```python
from build123d import *

# Parameters (mm, degrees)
F0_W     = 50.8
F0_H     = 431.8
F1_DEPTH = 25.4
F4_D     = 5.1054
F6_D     = 5.1054
F8_D     = 5.1054
F2_W     = 45.72
F2_H     = 20.32
F9_DEPTH = 431.8
F10_D    = 28.575


# Not quite as in the source:
# - a feature names something its author has since deleted; it is built from what else it names


with BuildPart() as f1:
    # F0 (on Top) → F1 (new body)
    with BuildSketch(Plane.XY):
        with Locations((-28.1036759261, 229.4025395081)):
            Rectangle(F0_W, F0_H)
    extrude(amount=F1_DEPTH)

    # F4 (through all)
    with Locations(Plane(origin=(-53.5036759261, 0, 0), x_dir=(0, -1, 0), z_dir=(-1, 0, 0))):
        with Locations((-26.2025395081, 12.7), (-331.0025395081, 12.7), (-381.8025395081, 12.7), (-356.4025395081, 12.7), (-407.2025395081, 12.7), (-178.6025395081, 12.7), (-229.4025395081, 12.7), (-204.0025395081, 12.7), (-280.2025395081, 12.7), (-254.8025395081, 12.7), (-305.6025395081, 12.7), (-102.4025395081, 12.7), (-153.2025395081, 12.7), (-51.6025395081, 12.7), (-127.8025395081, 12.7), (-77.0025395081, 12.7), (-432.6025395081, 12.7)):
            Hole(F4_D / 2)

    # F6 (through all)
    with Locations(Plane.XY.offset(25.4)):
        with Locations((-40.8036759261, 432.6025395081), (-15.4036759261, 432.6025395081), (-40.8036759261, 356.4025395081), (-40.8036759261, 381.8025395081), (-40.8036759261, 407.2025395081), (-40.8036759261, 254.8025395081), (-15.4036759261, 356.4025395081), (-15.4036759261, 254.8025395081), (-15.4036759261, 127.8025395081), (-40.8036759261, 102.4025395081), (-15.4036759261, 407.2025395081), (-15.4036759261, 331.0025395081), (-15.4036759261, 305.6025395081), (-40.8036759261, 204.0025395081), (-40.8036759261, 305.6025395081), (-15.4036759261, 280.2025395081), (-40.8036759261, 127.8025395081), (-15.4036759261, 381.8025395081), (-40.8036759261, 77.0025395081), (-40.8036759261, 178.6025395081), (-40.8036759261, 280.2025395081), (-15.4036759261, 77.0025395081), (-15.4036759261, 204.0025395081), (-15.4036759261, 178.6025395081), (-15.4036759261, 229.4025395081), (-15.4036759261, 153.2025395081), (-40.8036759261, 331.0025395081), (-40.8036759261, 229.4025395081), (-15.4036759261, 102.4025395081), (-40.8036759261, 153.2025395081)):
            Hole(F6_D / 2)

    # F8 (through all)
    with Locations(Plane.XY.offset(25.4)):
        with Locations((-45.6296759261, 56.4285395081), (-10.5776759261, 56.4285395081), (-10.5776759261, 21.3765395081), (-45.6296759261, 21.3765395081)):
            Hole(F8_D / 2)

    # F2 (on face) → F9 (cut)
    with BuildSketch(Plane(origin=(0, 445.3025395081, 0), x_dir=(-1, 0, 0), z_dir=(0, 1, 0))):
        with Locations((28.1036759261, 12.7)):
            Rectangle(F2_W, F2_H)
    extrude(amount=-F9_DEPTH, mode=Mode.SUBTRACT)

    # F10 (through all)
    with Locations(Plane.XY.offset(25.4)):
        with Locations((-28.1036759261, 38.9025395081)):
            Hole(F10_D / 2)


solid = f1.part
```
Here's how the part is built. I have some questions about the finished solid (model axes, mm). A direction names the side the tool comes from. Give positions to 0.01 mm unless a question says otherwise; leave off trailing zeros. Write each loop counter-clockwise with the first axis right and the second up, starting at its lowest first coordinate (ties: lowest second). Pieces come first, ordered by that corner, then holes.
(1) Imagine slicing it at B-B, the plane x = -34. Write out the boundary of the cut face in (y, z), and give its area (3 significant figures).
Output values:
outline: (13.5, 0) - (25.89, 0) - (25.89, 2.54) - (13.5, 2.54) - close; (13.5, 22.86) - (25.89, 22.86) - (25.89, 25.4) - (13.5, 25.4) - close; (51.92, 0) - (445.3, 0) - (445.3, 2.54) - (51.92, 2.54) - close; (51.92, 22.86) - (445.3, 22.86) - (445.3, 25.4) - (51.92, 25.4) - close
area: 2,060 mm2
(2) On a 3-axis mill with a long thin cutter (end or side, diameter ignored), from which of +Z, -Z, +X, -X, +Y, -Y can I reach the whole of each face in a straight line? I mean faces 4 (the face through (-53.504, 226, 13)), 5 (the face through (-50.964, 232.4, 12.6)). Say none if no direction works.
Output values:
face 4: +Z, -Z, -X, +Y, -Y
face 5: +Y, -Y
(3) If I drill on L1, parallel to X at y = 103, z = 23.5; L2, parallel to X at y = 222, z = 12.5; L3, parallel to Z at x = -24, y = 362, over which ranges is the centre line in solid material (lowest first)?
Output values:
L1: x = -53.5 to -43.29, -38.32 to -17.89, -12.92 to -2.7
L2: x = -53.5 to -50.96, -5.24 to -2.7
L3: z = 0 to 2.54, 22.86 to 25.4
(4) Thinking about a two-plate mould opening in X: for faces 1 (the face through (-28, 232, 25.4)), 2 (the face through (-2.704, 226, 13)), 3 (the face through (-28, 232, 22.86)), which applies, pulls with the +X half, pulls with the -X half, needs draft (parallel to the pull), parting line crosses it, or undercut?
Output values:
face 1: needs draft
face 2: pulls with the +X half
face 3: undercut
(5) Imagine slicing it at A-A, the plane y = 110. Write out the boundary of the cut face in (x, z).
Output values:
outline: (-53.5, 0) - (-2.7, 0) - (-2.7, 25.4) - (-53.5, 25.4) - close; hole (-50.96, 2.54) - (-5.24, 2.54) - (-5.24, 22.86) - (-50.96, 22.86) - close
